Geometry check sheet. Reference: drawing and pictorial views, mm from the part's lowest x, y, z. A direction names the side the tool comes from. Coordinates: 2 decimals unless noted, no trailing zeros. Loops run counter-clockwise (first coordinate to the right, second up) from the corner with the lowest first, then second, coordinate; pieces in that order, holes last. Notation, with made-up numbers: M 48.5,-16 L 99.5,-16 A25 ccw 99.5,-1 Z; hole C 35.25,5.25 d10. An arc over 180 degrees is marked long. Write each question's results on one line, items separated by ' | '. Start each with the question number.
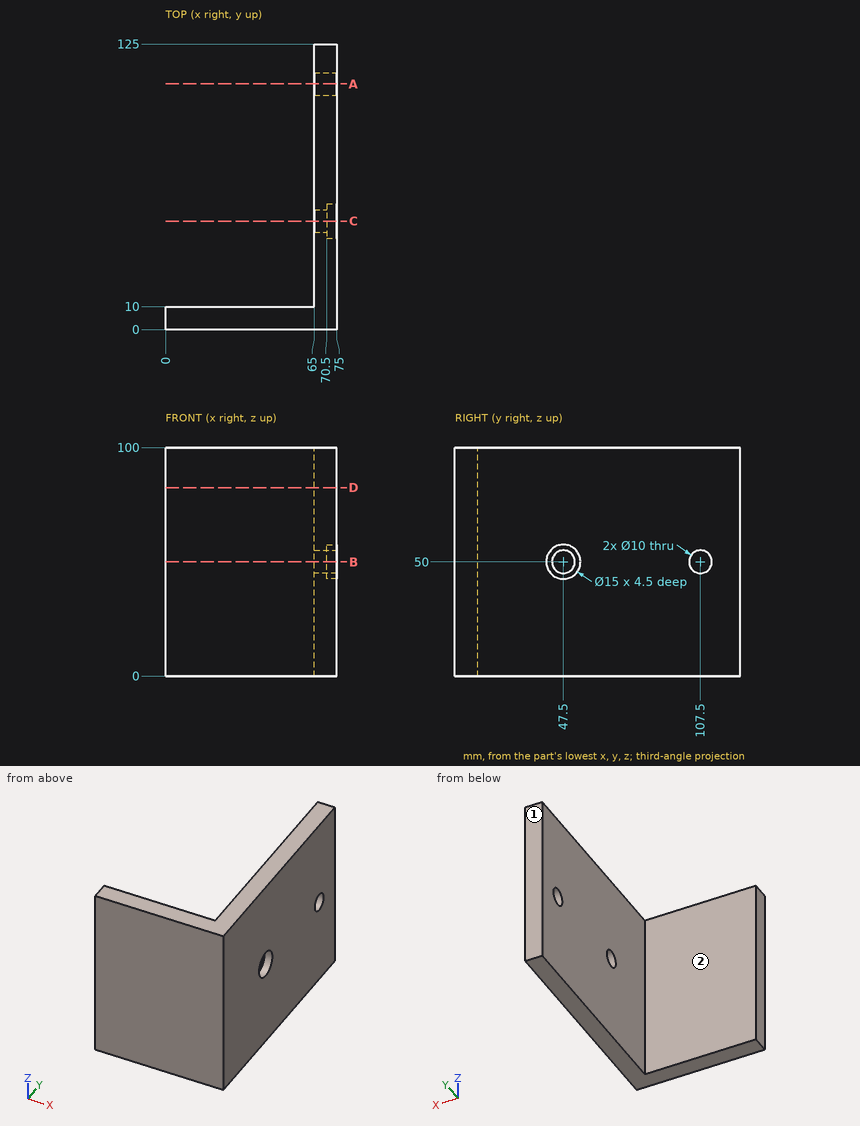
1) Gauge pin test, flat ends, axial feed: P1, Ø10, axis at x = 54, z = 41.5, coming from the +Y side; P2, Ø7.5, axis at y = 48, z = 47.5, coming from the +X side. Record the tip position at first contact, or that the pin passes through.
2) Section check C-C (y = 47.5). Enter the section's corners in (x, z), then the cut area to 4 significant figures.
3) Set-up check for the marked faces 1 and 2: record each of +Z, -Z, +X, -X, +Y, -Y from which the full face is reachable in a straight line by a thin tool's end or side.
4) Section check A-A (y = 107.5). Enter the section's corners in (x, z), then the cut area to 3 significant figures.
5) Section check B-B (z = 50). Enter the section's corners in (x, y), then the cut area to 3 significant figures.
6) Thickness scan on probe 1 along Y at (x, z) = (68, 50); probe 2 along Y at (x, z) = (72, 50); probe 3 along Z at (x, y) = (71, 47). Record the ranges inside material, lowest first.
7) Section check D-D (z = 82.5). Enter the section's corners in (x, y), then the cut area to 3 significant figures.
Return value:
1) P1: stops at y = 10 | P2: stops at x = 70.5
2) outline: M 65,0 L 75,0 L 75,42.5 L 70.5,42.5 L 70.5,45 L 65,45 Z; M 65,55 L 70.5,55 L 70.5,57.5 L 75,57.5 L 75,100 L 65,100 Z | area: 877.5 mm2
3) face 1: +Z, -Z, +X, -X, +Y | face 2: +Z, -Z, -X, +Y
4) outline: M 65,0 L 75,0 L 75,45 L 65,45 Z; M 65,55 L 75,55 L 75,100 L 65,100 Z | area: 900 mm2
5) outline: M 0,0 L 75,0 L 75,40 L 70.5,40 L 70.5,42.5 L 65,42.5 L 65,10 L 0,10 Z; M 65,52.5 L 70.5,52.5 L 70.5,55 L 75,55 L 75,102.5 L 65,102.5 Z; M 65,112.5 L 75,112.5 L 75,125 L 65,125 Z | area: 1,680 mm2
6) probe 1: y = 0 to 42.5, 52.5 to 102.5, 112.5 to 125 | probe 2: y = 0 to 40, 55 to 102.5, 112.5 to 125 | probe 3: z = 0 to 42.52, 57.48 to 100
7) outline: M 0,0 L 75,0 L 75,125 L 65,125 L 65,10 L 0,10 Z | area: 1,900 mm2
